Check sheet for the modelled part. Datum: model origin and axes. Units: mm. A direction names the side the tool comes from. Coordinates: 2 decimals unless noted, no trailing zeros. Write each loop counter-clockwise with the first axis right and the second up, starting at its lowest first coordinate (ties: lowest second). Pieces come first, ordered by that corner, then holes. Notation, with made-up numbers: (22, 20) - (28, 20) arc R11 ccw to (28, 38) - close; hole circle Ø8 at (-23, -7.5). An arc over 180 degrees is marked (long way). Use one line per item in the form item = value. Start each with the question number.
1. Cross-section at C-C on z = -8. Record the boundary of the cut face in (x, y) (3 decimals).
2. Cross-section at A-A on y = 0. Record the boundary of the cut face in (x, z) (3 decimals), then the cut area to 3 significant figures.
3. Tool access check on faces 1 (the face through (0, 0, 15.24)), 2 (the face through (-0.69, -3.1, 9.41)), 3 (the face through (-0.69, -3.1, -9.26)). Record the directions out of +Z, -Z, +X, -X, +Y, -Y that give a thin tool (end or side, any length) a straight path to the whole face; none if there is none.
4. Cross-section at D-D on z = -2. Record the boundary of the cut face in (x, y), then the cut area to 3 significant figures.
5. Go/stop test with flat-tipped pins: pin 1 Ø1.5 at (x, y) = (2, -3.5) entering from +Z; pin 2 Ø2 at (x, z) = (1, 11.5) entering from -Y (3 decimals); pin 3 Ø3 at (x, y) = (-5, -1.5) entering from -Z. Record where each tip stops, or that it passes through.
6. Scan lines: line 1 along Z through (x, y) = (0.25, 3.5); line 2 along X through (y, z) = (-1.5, 9.5); line 3 along Y through (x, z) = (5, -1.5). Record each from-to range of solid material in increasing order.
```python
from build123d import *

# Parameters (mm, degrees)
F0_R     = 3.175
F1_DEPTH = 15.24
F0_R_2   = 6.35
F2_DEPTH = 3.81
F3_SIZE  = 0.381


with BuildPart() as f1:
    # F0 (on Top) → F1 (new body, symmetric)
    with BuildSketch(Plane.XY):
        Circle(F0_R)
    extrude(amount=F1_DEPTH, both=True)

    # F0 (on Top) → F2 (join, symmetric)
    with BuildSketch(Plane.XY):
        Circle(F0_R_2)
        Circle(F0_R, mode=Mode.SUBTRACT)
    extrude(amount=F2_DEPTH, both=True)

    # F3
    f3_edges = [f1.edges().sort_by_distance(p)[0] for p in [
        (-6.35, 0, 3.81),
        (-6.35, 0, -3.81),
        (-3.175, 0, 15.24),
        (-3.175, 0, -15.24),
    ]]
    chamfer(f3_edges, length=F3_SIZE)


solid = f1.part
```
Final values:
q1.outline = circle Ø6.35 at (0, 0)
q2.outline = (-6.35, -3.429) - (-5.969, -3.81) - (-3.175, -3.81) - (-3.175, -14.859) - (-2.794, -15.24) - (2.794, -15.24) - (3.175, -14.859) - (3.175, -3.81) - (5.969, -3.81) - (6.35, -3.429) - (6.35, 3.429) - (5.969, 3.81) - (3.175, 3.81) - (3.175, 14.859) - (2.794, 15.24) - (-2.794, 15.24) - (-3.175, 14.859) - (-3.175, 3.81) - (-5.969, 3.81) - (-6.35, 3.429) - close
q2.area = 241 mm²
q3.face_1 = +Z, +X, -X, +Y, -Y
q3.face_2 = +Z
q3.face_3 = -Z
q4.outline = circle Ø12.7 at (0, 0)
q4.area = 127 mm²
q5.pin_1 = 3.81
q5.pin_2 = -3.175
q5.pin_3 = -3.81
q6.line_1 = -3.81 to 3.81
q6.line_2 = -2.8 to 2.8
q6.line_3 = -3.91 to 3.91
